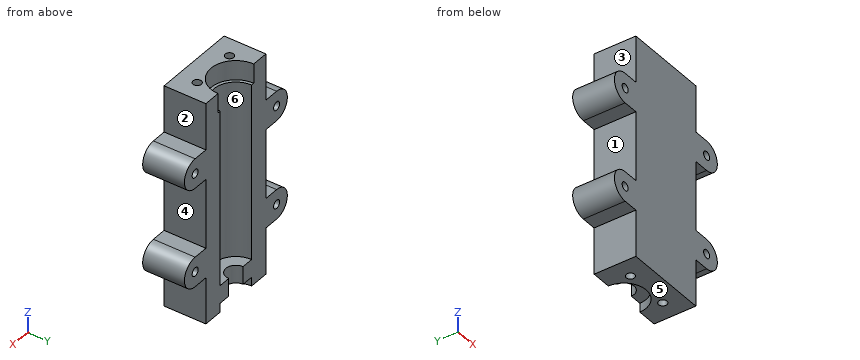
```python
from build123d import *

# Parameters (mm, degrees)
SKETCH_1_W               = 21
SKETCH_1_H               = 112
CUT_EXTRUDE_1_REACH      = 117.871
SKETCH_3_W               = 42
SKETCH_3_H               = 25
EXTRUDE_1_REACH          = 117.871
SKETCH_4_W               = 42
SKETCH_4_H               = 112
EXTRUDE_2_DEPTH          = 21
HOLE_WIZARD_M51_D        = 4.2
PATTERN_LINEAR_1_COUNT   = 2
PATTERN_LINEAR_1_PITCH   = 50
MIRROR_1_COPY_1_DEPTH    = 21
MIRROR_1_COPY_2_D        = 4.2
PATTERN_CIRCULAR_1_COUNT = 2
PATTERN_CIRCULAR_1_ANGLE = 90


with BuildPart() as part:
    # Эскиз1 → Повернуть1 (revolve)
    with BuildSketch(Plane(origin=(0, 0, 0), x_dir=(1, 0, 0), z_dir=(0, 1, 0))):
        with Locations((10.5, 56)):
            Rectangle(SKETCH_1_W, SKETCH_1_H)
    revolve(axis=Axis((0, 0, 0), (0, 0, -1)))

    # Эскиз2 → Вырез-Повернуть1 (revolve, cut)
    with BuildSketch(Plane(origin=(0, 0, 0), x_dir=(1, 0, 0), z_dir=(0, 1, 0)), mode=Mode.PRIVATE) as cut_revolve_1_sk:
        Polygon((0, 0), (12.5, 0), (12.5, 9.8), (11, 9.8), (11, 98.5), (5, 98.5), (5, 107.5), (11, 107.5), (11, 112), (0, 112), align=None)
    revolve(cut_revolve_1_sk.sketch.rotate(Axis((0, 0, -112), (0, 0, 1)), 180), axis=Axis((0, 0, -112), (0, 0, 1)), mode=Mode.SUBTRACT)

    # Вырез-Вытянуть1: up to this face of the body (flat: up to its plane)
    cut_extrude_1_end = Plane(part.part.faces().sort_by_distance((-20.406030304, 0, -112))[0])
    # Эскиз3 → Вырез-Вытянуть1 (cut, up to the picked face)
    with BuildSketch(Plane.XY, mode=Mode.PRIVATE) as cut_extrude_1_sk1:
        with Locations((0, 12.5)):
            Rectangle(SKETCH_3_W, SKETCH_3_H)
    cut_extrude_1_tool1 = split(extrude(cut_extrude_1_sk1.sketch, amount=-CUT_EXTRUDE_1_REACH, mode=Mode.PRIVATE), bisect_by=cut_extrude_1_end, keep=Keep.BOTH, mode=Mode.PRIVATE)
    add(cut_extrude_1_tool1.solids().sort_by(Axis((0, 12.5, 0), (0, 0, -1)))[0], mode=Mode.SUBTRACT)

    # Эскиз4 → Бобышка-Вытянуть1 (add, up to next)
    with BuildSketch(Plane(origin=(0, -21, 0), x_dir=(1, 0, 0), z_dir=(0, 1, 0)), mode=Mode.PRIVATE) as extrude_1_sk1:
        with Locations((0, 56)):
            Rectangle(SKETCH_4_W, SKETCH_4_H)
    extrude_1_tool1 = extrude(extrude_1_sk1.sketch, amount=EXTRUDE_1_REACH, mode=Mode.PRIVATE) - part.part
    add(extrude_1_tool1.solids().sort_by_distance((0, -21, -56))[0])
    add(extrude_1_tool1.solids().sort_by_distance((0, -21, -56))[1])

    # Эскиз5 → Бобышка-Вытянуть2 (add)
    with BuildSketch(Plane(origin=(0, -21, 0), x_dir=(1, 0, 0), z_dir=(0, 1, 0))):
        with BuildLine():
            Line((21, 23.5), (28.5, 23.5))
            ThreePointArc((28.5, 23.5), (36, 31), (28.5, 38.5))
            Line((28.5, 38.5), (21, 38.5))
            Line((21, 38.5), (21, 23.5))
        make_face()
    extrude_2 = extrude(amount=EXTRUDE_2_DEPTH)

    # Сверление под метчик M51 (through all)
    with Locations(Plane(origin=(28.5, 0, -31), x_dir=(0, 0, 1), z_dir=(0, 1, 0))):
        with Locations((0, 0)):
            hole_wizard_m51 = Hole(HOLE_WIZARD_M51_D / 2)

    # Линейный массив1: Бобышка-Вытянуть2, Сверление под метчик M51 ×2
    with Locations(*[(0, 0, -i * PATTERN_LINEAR_1_PITCH) for i in range(1, PATTERN_LINEAR_1_COUNT)]):
        add(extrude_2)
        add(hole_wizard_m51, mode=Mode.SUBTRACT)

    # Зеркальное отражение1: Бобышка-Вытянуть2, Сверление под метчик M51 across plane
    add(extrude_2.mirror(Plane(origin=(0, 0, 0), x_dir=(0, 0, 1), z_dir=(1, 0, 0))))
    add(hole_wizard_m51.mirror(Plane(origin=(0, 0, 0), x_dir=(0, 0, 1), z_dir=(1, 0, 0))), mode=Mode.SUBTRACT)

    # Зеркальное отражение1 copy 1 sketch → Зеркальное отражение1 copy 1 (add)
    with BuildSketch(Plane(origin=(0, -21, -50), x_dir=(-1, 0, 0), z_dir=(0, 1, 0))):
        with BuildLine():
            Line((21, -23.5), (28.5, -23.5))
            ThreePointArc((28.5, -23.5), (36, -31), (28.5, -38.5))
            Line((28.5, -38.5), (21, -38.5))
            Line((21, -38.5), (21, -23.5))
        make_face()
    extrude(amount=MIRROR_1_COPY_1_DEPTH)

    # Зеркальное отражение1 copy 2 (through all)
    with Locations(Plane(origin=(-28.5, 0, -81), x_dir=(0, 0, 1), z_dir=(0, 1, 0))):
        with Locations((0, 0)):
            Hole(MIRROR_1_COPY_2_D / 2)

    # Эскиз8 → Сверление под метчик M52 (revolve, cut)
    with BuildSketch(Plane(origin=(11.313708499, -11.313708499, 0), x_dir=(0, -1, 0), z_dir=(1, 0, 0))):
        Polygon((0, 0), (0, 26.2618073), (2.1, 25), (2.1, 0), align=None)
    hole_wizard_m52 = revolve(axis=Axis((11.313708499, -11.313708499, 6.35), (0, 0, -1)), mode=Mode.SUBTRACT)

    # Круговой массив1: Сверление под метчик M52 ×2 about axis
    pattern_circular_1_axis = Axis((0, 0, 0), (0, 0, -1))
    for i in range(1, PATTERN_CIRCULAR_1_COUNT):
        add(hole_wizard_m52.rotate(pattern_circular_1_axis, i * PATTERN_CIRCULAR_1_ANGLE / (PATTERN_CIRCULAR_1_COUNT - 1)), mode=Mode.SUBTRACT)

    # Зеркальное отражение2: Сверление под метчик M52 across plane
    add(hole_wizard_m52.mirror(Plane.XY.offset(-56)), mode=Mode.SUBTRACT)

    # Зеркальное отражение2 copy 1 sketch → Зеркальное отражение2 copy 1 (revolve, cut)
    with BuildSketch(Plane(origin=(-11.313708499, -11.313708499, -112), x_dir=(-1, 0, 0), z_dir=(0, -1, 0))):
        Polygon((0, 0), (0, -26.2618073), (2.1, -25), (2.1, 0), align=None)
    revolve(axis=Axis((-11.313708499, -11.313708499, -118.35), (0, 0, -1)), mode=Mode.SUBTRACT)


solid = part.part
```
Source: CAD feature listing. Evaluate the final solid. Frame: model axes, mm. Face numbers are marked on the shaded views. A direction names the side the tool comes from. Give positions to 0.01 mm unless a question says otherwise; leave off trailing zeros. Loops run counter-clockwise (first coordinate to the right, second up) from the corner with the lowest first, then second, coordinate; pieces in that order, holes last. Notation, with made-up numbers: (73.25, 60) - (85.25, 60) arc R7 ccw to (85.25, 69) - close; hole circle Ø5 at (38, -4). An arc over 180 degrees is marked (long way). Use CSV: the item, a comma, the result in double quotes. Start each with the question number.
1. Section B-B (x = 0). Output: boundary loops of the cut face in (y, z).
2. Section A-A (z = -31). Output: boundary loops of the cut face in (x, y).
3. Pin query (flat end, axial travel): pin 1 (4 mm diameter, centred on x = 28.5, z = -31, fed in from -Y); pin 2 (10.5 mm diameter, centred on y = -14.5, z = -101.5, fed in from -X); pin 3 (8 mm diameter, centred on x = -23.5, y = -10, fed in from +Z); pin 4 (2 mm diameter, centred on x = -26.5, y = -9.5, fed in from -Z). Return the tip coordinate at first contact, or that it passes through.
4. Reachability of the marked faces 1, 2 and 3 from +Z, -Z, +X, -X, +Y, -Y: full face, straight path, thin tool, end or side. Return the list, or none.
5. Draft query along X for the marked faces 4, 5 and 6. Return one class per face: +X half, -X half, draft (parallel to the pull), parting line (faces both ways), or undercut.
6. Section D-D (z = -67.5). Output: boundary loops of the cut face in (x, y), then the cut area to 3 significant figures.
7. Section C-C (y = -3.25). Count the separate pieces of the cut face and the enclosed holes in it, then the cut area to 3 significant figures.
8. Ray query, L1, parallel to X at y = -11.5, z = -31; L2, parallel to X at y = -18.5, z = -30.5; L3, parallel to Z at x = 23, y = -18.5. Return the intervals inside material, ascending.
Response:
1,outline,"(-21, -112) - (-11, -112) - (-11, -107.5) - (-5, -107.5) - (-5, -98.5) - (-11, -98.5) - (-11, -9.8) - (-12.5, -9.8) - (-12.5, 0) - (-21, 0) - close"
2,outline,"(-36, -21) - (-30.6, -21) - (-30.6, 0) - (-36, 0) - close; (-26.4, -21) - (26.4, -21) - (26.4, 0) - (11, 0) arc R11 cw to (-11, 0) - (-26.4, 0) - close; (30.6, -21) - (36, -21) - (36, 0) - (30.6, 0) - close"
3,pin 1,"through"
3,pin 2,"x = -21"
3,pin 3,"z = 0"
3,pin 4,"z = -88.5"
4,face 1,"-X, +Y, -Y"
4,face 2,"+Z, +X, +Y, -Y"
4,face 3,"+Z, -X, +Y, -Y"
5,face 4,"+X half"
5,face 5,"draft"
5,face 6,"undercut"
6,outline,"(-21, -21) - (21, -21) - (21, 0) - (11, 0) arc R11 cw to (-11, 0) - (-21, 0) - close"
6,area,"692 mm²"
7,separate pieces,"2"
7,enclosed holes,"4"
7,area,"3,190 mm²"
8,L1,"-36 to -30.6, -26.4 to 26.4, 30.6 to 36"
8,L2,"-35.98 to -30.54, -26.46 to 26.46, 30.54 to 35.98"
8,L3,"-88.5 to -73.5, -38.5 to -23.5"
